from build123d import *

# Parameters (mm, degrees)
F0_W     = 98
F0_H     = 90
F1_DEPTH = 1.6
F2_R     = 2
F3_DEPTH = 25
F4_W     = 40
F4_H     = 5
F5_DEPTH = 14


with BuildPart() as f1:
    # F0 (on Front) → F1 (new body)
    with BuildSketch(Plane.XZ):
        Rectangle(F0_W, F0_H)
    extrude(amount=F1_DEPTH)

    # F2 (on face) → F3 (cut)
    with BuildSketch(Plane.XZ.offset(1.6)):
        with Locations((-46, 39)):
            Circle(F2_R)
        with Locations((-46, 19)):
            Circle(F2_R)
        with Locations((7, 19)):
            Circle(F2_R)
        with Locations((45, 39)):
            Circle(F2_R)
        with Locations((-46, -22)):
            Circle(F2_R)
        with Locations((7, -22)):
            Circle(F2_R)
        with Locations((45, -22)):
            Circle(F2_R)
    extrude(amount=-F3_DEPTH, mode=Mode.SUBTRACT)

    # F4 (on face) → F5 (join)
    with BuildSketch(Plane(origin=(0, 0, 0), x_dir=(-1, 0, 0), z_dir=(0, 1, 0))):
        with Locations((19.5, 18.5)):
            Rectangle(F4_W, F4_H)
        with Locations((19.5, -22.5)):
            Rectangle(F4_W, F4_H)
    extrude(amount=F5_DEPTH)


solid = f1.part
Could you check a few things on this model? Use its own coordinates, in mm. A direction names the side the tool comes from. Coordinates: 2 decimals unless noted, no trailing zeros. Order: outer loops, then holes, each group sorted by start corner. A loop starts at its lowest first (then second) coordinate and runs counter-clockwise, first axis right, second up. Notation, with made-up numbers: (-23.5, -14) -> (-4.5, -14) arc R18 ccw to (-4.5, 16) -> close; hole circle Ø1 at (82, 72.25). An arc over 180 degrees is marked (long way). One line per item, written item: value. Start each with the question number.
1) We'd pull the mould along X, two halves only. Please class faces 1 (the flat face through (-19, 7, 21)), 2 (the flat face through (-39.5, 7, 18)), 3 (the cylindrical face through (45, -1, 37)), 4 (the flat face through (0.5, 7, -23)): +X half, -X half, draft (parallel to the pull), parting line (faces both ways), or undercut.
2) I'm going to push flat-ended pins straight in: pin 1 (1 mm diameter, centred on x = 22.5, z = 5, fed in from +Y); pin 2 (3.5 mm diameter, centred on x = 45, z = 39, fed in from +Y); pin 3 (8 mm diameter, centred on y = 8, z = -26, fed in from -X); pin 4 (4 mm diameter, centred on y = 7.5, z = 17.5, fed in from +X). Where does each tip first touch, or does it pass through?
3) Imagine slicing it at D-D on x = 7. List the corners of the cut face in (y, z) for me.
4) Imagine slicing it at A-A on z = 39. List the corners of the cut face in (x, y) for me.
5) Which directions (+Z, -Z, +X, -X, +Y, -Y) give clear straight access to the entire face, cutting with the end or side of a thin tool? Please do faces 5 (the flat face through (-19, 7, -25)), 6 (the flat face through (-39.5, 7, -23)), 7 (the flat face through (0.5, 7, 18)), 8 (the flat face through (-19, 7, -20)).
6) Imagine slicing it at B-B on y = 11.75. List the corners of the cut face in (x, z) for me.
7) Imagine slicing it at C-C on x = -46. List the corners of the cut face in (y, z) for me, plus the area to 3 significant figures.
8) If I drill on L1, parallel to Z at x = -46, y = -0.7; L2, parallel to Z at x = 45, y = -0.45; L3, parallel to Z at x = 7, y = -0.55, over which ranges is the centre line in solid material (lowest first)? Write a range as [from, to].
Answer list:
1. face 1: draft
1. face 2: -X half
1. face 3: undercut
1. face 4: +X half
2. pin 1: stops at y = 0
2. pin 2: passes through
2. pin 3: stops at x = -39.5
2. pin 4: stops at x = 0.5
3. outline: (-1.6, -45) -> (0, -45) -> (0, -24) -> (-1.6, -24) -> close; (-1.6, -20) -> (0, -20) -> (0, 17) -> (-1.6, 17) -> close; (-1.6, 21) -> (0, 21) -> (0, 45) -> (-1.6, 45) -> close
4. outline: (-49, -1.6) -> (-48, -1.6) -> (-48, 0) -> (-49, 0) -> close; (-44, -1.6) -> (43, -1.6) -> (43, 0) -> (-44, 0) -> close; (47, -1.6) -> (49, -1.6) -> (49, 0) -> (47, 0) -> close
5. face 5: -Z, +X, -X, +Y
5. face 6: +Z, -Z, -X, +Y
5. face 7: +Z, -Z, +X, +Y
5. face 8: +X, -X, +Y
6. outline: (-39.5, -25) -> (0.5, -25) -> (0.5, -20) -> (-39.5, -20) -> close; (-39.5, 16) -> (0.5, 16) -> (0.5, 21) -> (-39.5, 21) -> close
7. outline: (-1.6, -45) -> (0, -45) -> (0, -24) -> (-1.6, -24) -> close; (-1.6, -20) -> (0, -20) -> (0, 17) -> (-1.6, 17) -> close; (-1.6, 21) -> (0, 21) -> (0, 37) -> (-1.6, 37) -> close; (-1.6, 41) -> (0, 41) -> (0, 45) -> (-1.6, 45) -> close
7. area: 125 mm2
8. L1: z = [-45, -24], [-20, 17], [21, 37], [41, 45]
8. L2: z = [-45, -24], [-20, 37], [41, 45]
8. L3: z = [-45, -24], [-20, 17], [21, 45]
